from build123d import *

# Parameters (mm, degrees)
F0_R     = 3.1
F0_R_2   = 1.5
F1_DEPTH = 4.3
F3_DEPTH = 8
F4_R     = 1
F5_DEPTH = 8
F6_DEPTH = 6


with BuildPart() as f1:
    # F0 (on Top) → F1 (new body)
    with BuildSketch(Plane.XY):
        Circle(F0_R)
        Circle(F0_R_2, mode=Mode.SUBTRACT)
        Circle(F0_R_2)
    extrude(amount=F1_DEPTH)

    # F2 (on face) → F3 (join)
    with BuildSketch(Plane.XY.offset(4.3)):
        with BuildLine():
            Line((2.164151, -1.529363), (2.164151, 1.529363))
            ThreePointArc((2.164151, 1.529363), (0, 2.65), (-2.164151, 1.529363))
            Line((-2.164151, 1.529363), (-2.164151, -1.529363))
            ThreePointArc((-2.164151, -1.529363), (0, -2.65), (2.164151, -1.529363))
        make_face()
    extrude(amount=F3_DEPTH)

    # F4 (on face) → F5 (cut)
    with BuildSketch(Plane.XY.offset(12.3)):
        Circle(F4_R)
    extrude(amount=-F5_DEPTH, mode=Mode.SUBTRACT)

    # F0 (on Top) → F6 (cut)
    with BuildSketch(Plane.XY):
        Circle(F0_R_2)
    extrude(amount=F6_DEPTH, mode=Mode.SUBTRACT)


solid = f1.part
Part model, mm, in its own coordinate system. A direction names the side the tool comes from. Give positions to 0.01 mm unless a question says otherwise; leave off trailing zeros. Order: outer loops, then holes, each group sorted by start corner. A loop starts at its lowest first (then second) coordinate and runs counter-clockwise, first axis right, second up. Notation, with made-up numbers: (7.25, -16) - (28.25, -16) arc R28 cw to (28.25, 14) - close; hole circle Ø9 at (75.5, -21.75). An arc over 180 degrees is marked (long way). Use a Markdown table: item, result.
1) Two-plate mould, pull along Y, no slides. Class faces 3 (the cylindrical face through (0.04, 2.65, 8.24)), 4 (the flat face through (2.164, 0, 8)), 5 (the cylindrical face through (-1.5, 0.07, 2.96)), 6 (the cylindrical face through (-0.04, -2.65, 8.24)): +Y half, -Y half, draft (parallel to the pull), parting line (faces both ways), or undercut.
Checked values:
| item | result |
|---|---|
| face 3 | +Y half |
| face 4 | draft |
| face 5 | undercut |
| face 6 | -Y half |
2) Saw through at B-B on z = 11. List the corners of the cut face in (x, y).
Checked values:
| item | result |
|---|---|
| outline | (-2.16, -1.53) arc R2.65 ccw to (2.16, -1.53) - (2.16, 1.53) arc R2.65 ccw to (-2.16, 1.53) - close; hole circle Ø2 at (0, 0) |
3) Saw through at A-A on x = 0. List the corners of the cut face in (y, z), plus the area to 3 significant figures.
Checked values:
| item | result |
|---|---|
| outline | (-3.1, 0) - (-1.5, 0) - (-1.5, 6) - (-1, 6) - (-1, 12.3) - (-2.65, 12.3) - (-2.65, 4.3) - (-3.1, 4.3) - close; (1, 6) - (1.5, 6) - (1.5, 0) - (3.1, 0) - (3.1, 4.3) - (2.65, 4.3) - (2.65, 12.3) - (1, 12.3) - close |
| area | 38.5 mm² |
4) Saw through at C-C on y = -0.5. List the corners of the cut face in (x, z).
Checked values:
| item | result |
|---|---|
| outline | (-3.06, 0) - (-1.41, 0) - (-1.41, 6) - (-0.87, 6) - (-0.87, 12.3) - (-2.16, 12.3) - (-2.16, 4.3) - (-3.06, 4.3) - close; (0.87, 6) - (1.41, 6) - (1.41, 0) - (3.06, 0) - (3.06, 4.3) - (2.16, 4.3) - (2.16, 12.3) - (0.87, 12.3) - close |
5) Flat gauge pins, fed straight in: P1, Ø2.5, axis at y = 0, z = 9.5, coming from the +X side; P2, Ø1.5, axis at y = 0.5, z = 10, coming from the -X side; P3, Ø1.8, axis at x = 0, y = 0, coming from the +Z side; P4, Ø2.5, axis at x = 0, y = 0, coming from the -Z side. Where does each tip first touch, or does it go through?
Checked values:
| item | result |
|---|---|
| P1 | x = 2.16 |
| P2 | x = -2.16 |
| P3 | through |
| P4 | z = 6 |
6) Probe L1, parallel to Z at x = -2.5, y = -1.5; L2, parallel to Y at x = 0, z = 3.6; L3, parallel to X at y = 1.5, z = 7. List the from-to ranges inside material, lowest first. Write a range as from..to.
Checked values:
| item | result |
|---|---|
| L1 | 0..4.3 |
| L2 | -3.1..-1.5, 1.5..3.1 |
| L3 | -2.16..2.16 |
7) Saw through at D-D on y = 1.25. List the corners of the cut face in (x, z), plus the area to 3 significant figures.
Checked values:
| item | result |
|---|---|
| outline | (-2.84, 0) - (-0.83, 0) - (-0.83, 6) - (0.83, 6) - (0.83, 0) - (2.84, 0) - (2.84, 4.3) - (2.16, 4.3) - (2.16, 12.3) - (-2.16, 12.3) - (-2.16, 4.3) - (-2.84, 4.3) - close |
| area | 49.1 mm² |
8) 3-axis set-ups, long thin cutter, end or side, ignore diameter. For faces 1 (the flat face through (-2.164, 0, 8)), 2 (the flat face through (1, -1, 12.3)): which of +Z, -Z, +X, -X, +Y, -Y reach the whole face in a straight line?
Checked values:
| item | result |
|---|---|
| face 1 | +Z, -X, +Y, -Y |
| face 2 | +Z, +X, -X, +Y, -Y |
